Autodesk Inventor part; units mm, degrees
ref_plane "YZ Plane" through (0, 0, 0) normal (1, 0, 0) x (0, 1, 0)
ref_plane "XZ Plane" through (0, 0, 0) normal (0, 1, 0) x (-1, 0, 0)
ref_plane "XY Plane" through (0, 0, 0) normal (0, 0, 1) x (1, 0, 0)
sketch "Sketch1" plane through (0, 0, 0) normal (0, 1, 0) x (-1, 0, 0)
  line L0 (11.5, 6.25) -> (-11.5, 6.25)
  line L1 (-11.5, 6.25) -> (-11.5, -6.25)
  line L2 (-11.5, -6.25) -> (11.5, -6.25)
  line L3 (11.5, -6.25) -> (11.5, 6.25)
  line L4 (11.5, 6.25) -> (-11.5, -6.25) construction
  line L5 (-11.5, 6.25) -> (11.5, -6.25) construction
  line L6 (17, 8.5) -> (-17, 8.5)
  line L7 (-17, 8.5) -> (-17, -8.5)
  line L8 (-17, -8.5) -> (17, -8.5)
  line L9 (17, -8.5) -> (17, 8.5) construction
  line L10 (17, 8.5) -> (-17, -8.5) construction
  line L11 (-17, 8.5) -> (17, -8.5) construction
  line L12 (38.8, 0) -> (-26.3, 0)
  line L13 (0, -20.3) -> (0, 20.3)
  line L14 (29.5, 14.5) -> (18.5, 14.5)
  line L15 (18.5, 14.5) -> (18.5, -14.5) construction
  line L16 (18.5, -14.5) -> (29.5, -14.5)
  line L17 (29.5, -14.5) -> (29.5, 14.5)
  line L18 (29.5, 14.5) -> (18.5, -14.5) construction
  line L19 (18.5, 14.5) -> (29.5, -14.5) construction
  line L20 (18.5, 14.5) -> (17, 8.5)
  line L21 (17, -8.5) -> (18.5, -14.5)
  circle A0 centre (-14, 0) radius 1
  circle A1 centre (14, 0) radius 1
  circle A2 centre (24, 9.25) radius 1.25
  circle A3 centre (24, -9.25) radius 1.25
  point P0 (0, 0)
  point P1 (24, 0)
  dimension "d0" = 23
  dimension "d1" = 12.5
  dimension "d2" = 17
  dimension "d3" = 34
  dimension "d11" = 2
  dimension "d12" = 28
  dimension "d13" = 12.5
  dimension "d14" = 2.5
  dimension "d15" = 9.25
  dimension "d16" = 29
  dimension "d18" = 5.5
extrude "Extrusion1" add sketch "Sketch1" along normal blind 4 contours L0 L13 L6 L20 L14 L17 L12 A1 L3 | L0 L1 L12 A0 L7 L6 L13 | L12 A1 L17 L16 L21 L8 L13 L2 L3 | L1 L2 L13 L8 L7 L12 A0
sketch "Sketch2" plane through (0, 4, 0) normal (0, 1, 0) x (1, 0, 0)
  circle A0 centre (14, 0) radius 1
  circle A1 centre (14, 0) radius 2
  line L0 (0, 20.3) -> (0, -20.3)
  circle A2 centre (-14, 0) radius 2
  point P0 (0, 0)
  dimension "d21" = 4
extrude "Extrusion2" cut sketch "Sketch2" against normal blind 2
sketch "Sketch3" plane through (0, 0, 0) normal (0, -1, 0) x (1, 0, 0)
  line L0 (-38.8, 0) -> (26.3, 0)
  circle A0 centre (-24, 9.25) radius 1.25
  circle A1 centre (-24, 9.25) radius 2
  circle A2 centre (-24, -9.25) radius 2
  point P0 (0, 0)
  dimension "d24" = 4
extrude "Extrusion3" cut sketch "Sketch3" against normal blind 2 contours A0 | A1 | A2
fillet "Fillet1" radius 5 8 edges at (-18.5, 2, 14.5) (-17, 2, 8.5) (-29.5, 2, 14.5) (-29.5, 2, -14.5) (-18.5, 2, -14.5) (-17, 2, -8.5) (17, 2, -8.5) (17, 2, 8.5)
properties part number "mount1"
Part model, mm, in its own coordinate system. A direction names the side the tool comes from. Round coordinates to 2 decimals unless told otherwise and drop trailing zeros. Write each loop counter-clockwise with the first axis right and the second up, starting at its lowest first coordinate (ties: lowest second). Pieces come first, ordered by that corner, then holes. Notation, with made-up numbers: (-37, 35) -> (-14, 35) arc R21 cw to (-14, 51) -> close; hole circle Ø2 at (39, 28). An arc over 180 degrees is marked (long way). Return JSON: item names as keys, results as strings. Group by question number.
Q1. Pin check, flat tips, straight feed: pin 1 (1.2 mm diameter, centred on x = -2, y = 1.5, fed in from -Z); pin 2 (2 mm diameter, centred on x = -20.5, y = 0.5, fed in from -Z); pin 3 (1.2 mm diameter, centred on x = -14, z = -0.5, fed in from +Y). Stop position of each tip, or through.
Q2. Saw through at C-C on x = -24. Write the cut outline in (y, z).
Q3. Probe L1, parallel to Z at x = -24, y = 1.45; L2, parallel to X at y = 3, z = 0; L3, parallel to X at y = 3.8, z = 3.75. List the from-to ranges inside material, lowest first. Write a range as [from, to].
Q4. Saw through at B-B on x = 1. Write the cut outline in (y, z).
Q5. Which spindle directions (+Z, -Z, +X, -X, +Y, -Y) get a long thin tool onto all of the face, cutting with end or side? Do faces 4 (the flat face through (15, 2, 1)), 5 (the flat face through (0, 2, -6.25)), 6 (the flat face through (-23, 2, 14.5)), 7 (the flat face through (-25, 2, 8)). Say none if no direction does.
Q6. Saw through at A-A on z = 0. Write the cut outline in (x, y).
Q7. Mould opens along X. For faces 1 (the cylindrical face through (15.5, 2.03, 7.07)), 2 (the flat face through (-29.5, 2, 0)), 3 (the cylindrical face through (-15, 1, 0)) say: pulls with the +X half, pulls with the -X half, needs draft (parallel to the pull), parting line crosses it, or undercut.
Q8. Saw through at D-D on z = -4.75. Write the cut outline in (x, y), plus the area to 3 significant figures.
Answer:
{
 "1": {"pin 1": "z = -8.5", "pin 2": "z = -14.44", "pin 3": "y = 2"},
 "2": {"outline": "(0, -14.5) -> (4, -14.5) -> (4, -10.5) -> (2, -10.5) -> (2, -11.25) -> (0, -11.25) -> close; (0, -7.25) -> (2, -7.25) -> (2, -8) -> (4, -8) -> (4, 8) -> (2, 8) -> (2, 7.25) -> (0, 7.25) -> close; (0, 11.25) -> (2, 11.25) -> (2, 10.5) -> (4, 10.5) -> (4, 14.5) -> (0, 14.5) -> close"},
 "3": {"L1": "[-14.5, -11.25], [-7.25, 7.25], [11.25, 14.5]", "L2": "[-29.5, -16], [-12, -11.5], [11.5, 12], [16, 17]", "L3": "[-29.5, -11.5], [11.5, 16.99]"},
 "4": {"outline": "(0, -8.5) -> (4, -8.5) -> (4, -6.25) -> (0, -6.25) -> close; (0, 6.25) -> (4, 6.25) -> (4, 8.5) -> (0, 8.5) -> close"},
 "5": {"face 4": "+Y", "face 5": "+Y, -Y", "face 6": "+Z, +X, -X, +Y, -Y", "face 7": "-Y"},
 "6": {"outline": "(-29.5, 0) -> (-15, 0) -> (-15, 2) -> (-16, 2) -> (-16, 4) -> (-29.5, 4) -> close; (-13, 0) -> (-11.5, 0) -> (-11.5, 4) -> (-12, 4) -> (-12, 2) -> (-13, 2) -> close; (11.5, 0) -> (13, 0) -> (13, 2) -> (12, 2) -> (12, 4) -> (11.5, 4) -> close; (15, 0) -> (17, 0) -> (17, 4) -> (16, 4) -> (16, 2) -> (15, 2) -> close"},
 "7": {"face 1": "pulls with the +X half", "face 2": "pulls with the -X half", "face 3": "undercut"},
 "8": {"outline": "(-29.5, 0) -> (-11.5, 0) -> (-11.5, 4) -> (-29.5, 4) -> close; (11.5, 0) -> (16.84, 0) -> (16.84, 4) -> (11.5, 4) -> close", "area": "93.4 mm2"}
}
